Here's the drawing with two shaded views (mm, measured from the low corner). I have some questions. Coordinates: 2 decimals unless noted, no trailing zeros. Write each loop counter-clockwise with the first axis right and the second up, starting at its lowest first coordinate (ties: lowest second). Pieces come first, ordered by that corner, then holes.
Item 1: If we section it at A-A (x = 110): Please give me the cut outline in (y, z), then the cut area to 3 significant figures.
Item 2: If we section it at C-C (y = 6): Please give me the cut outline in (x, z), then the cut area to 3 significant figures.
Item 3: If we section it at D-D (z = 198): Please give me the cut outline in (x, y).
Item 4: If I drill on line 1 (X direction, y = 7, z = 110); line 2 (X direction, y = 18.4, z = 110); line 3 (Y direction, x = 100, z = 28.5), over which ranges is the centre line in solid material (lowest first)?
Item 5: We'd pull the mould along X, two halves only. Please class the marked faces 1, 2 and 3: +X half, -X half, draft (parallel to the pull), parting line (faces both ways), or undercut.
Item 6: I'm going to push flat-ended pins straight in: pin 1 Ø4 at (x, y) = (91.5, 51.5) entering from -Z; pin 2 Ø12 at (x, y) = (169, 21.5) entering from -Z; pin 3 Ø10 at (y, z) = (45.5, 38.5) entering from +X. Where does each tip first touch, or does it pass through?
Item 7: If we section it at B-B (z = 110): Please give me the cut outline in (x, y), then the cut area to 3 significant figures.
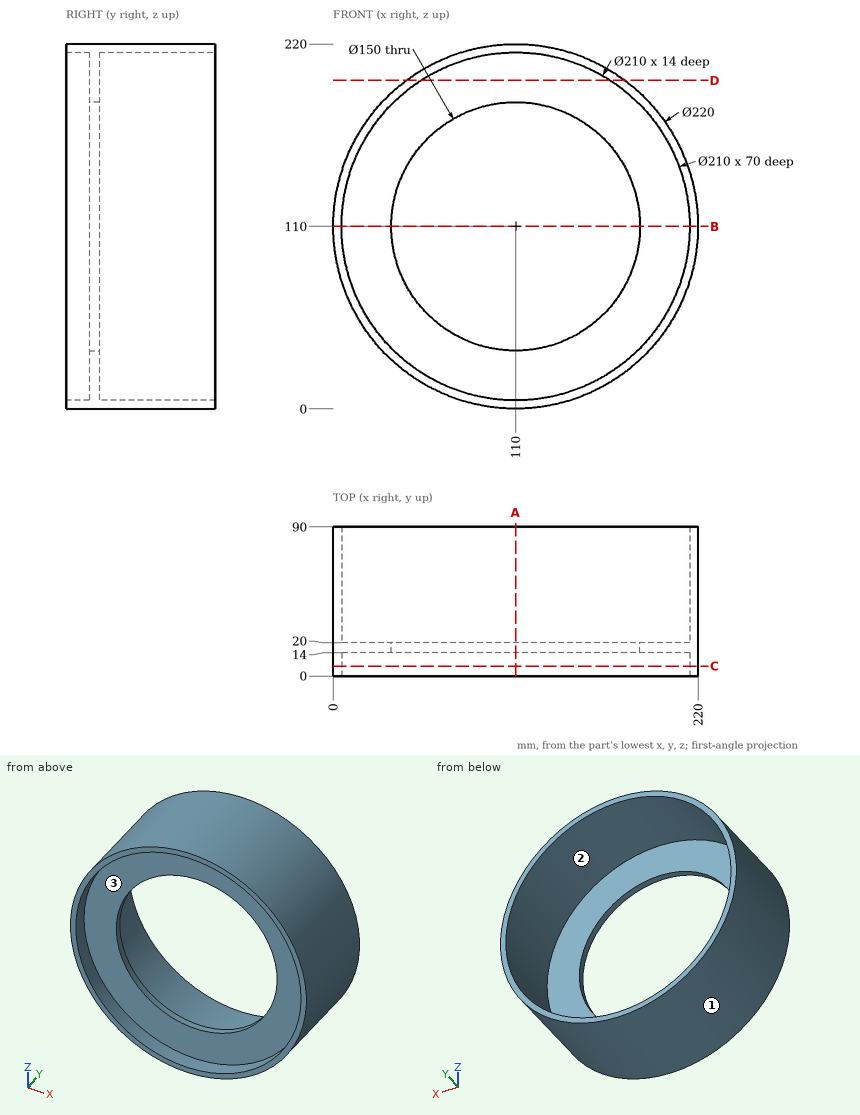
Answer list:
1. outline: (0, 0) - (90, 0) - (90, 5) - (20, 5) - (20, 35) - (14, 35) - (14, 5) - (0, 5) - close; (0, 215) - (14, 215) - (14, 185) - (20, 185) - (20, 215) - (90, 215) - (90, 220) - (0, 220) - close
1. area: 1,260 mm2
2. outline: circle Ø220 at (110, 110); hole circle Ø210 at (110, 110)
2. area: 3,380 mm2
3. outline: (44, 0) - (52.72, 0) - (52.72, 14) - (167.28, 14) - (167.28, 0) - (176, 0) - (176, 90) - (167.28, 90) - (167.28, 20) - (52.72, 20) - (52.72, 90) - (44, 90) - close
4. line 1: x = 0 to 5, 215 to 220
4. line 2: x = 0 to 35, 185 to 220
4. line 3: y = 14 to 20
5. face 1: parting line
5. face 2: undercut
5. face 3: undercut
6. pin 1: stops at z = 1.24
6. pin 2: stops at z = 13.61
6. pin 3: stops at x = 197.62
7. outline: (0, 0) - (5, 0) - (5, 14) - (35, 14) - (35, 20) - (5, 20) - (5, 90) - (0, 90) - close; (185, 14) - (215, 14) - (215, 0) - (220, 0) - (220, 90) - (215, 90) - (215, 20) - (185, 20) - close
7. area: 1,260 mm2
